Read the model definition and answer for the solid it produces. Units are mm, in the model's axes. Coordinates: 2 decimals unless noted, no trailing zeros. Loops run counter-clockwise (first coordinate to the right, second up) from the corner with the lowest first, then second, coordinate; pieces in that order, holes last.
from build123d import *

# Parameters (mm, degrees)
F0_R           = 12
F1_DEPTH       = 5
F2_R           = 21
F3_DEPTH       = 12.001
F3_DEPTH_BACK  = 12.001
F4_R           = 10.5
F5_DEPTH       = 6
F5_DEPTH_BACK  = 4
F6_SIZE        = 2
F8_D           = 4.5
F8_CSINK_D     = 10
F8_CSINK_ANGLE = 90


with BuildPart() as f1:
    # F0 (on Right) → F1 (new body)
    with BuildSketch(Plane.YZ):
        Circle(F0_R)
    extrude(amount=F1_DEPTH)

    # F2 (on Top) → F3 (cut, two sides)
    with BuildSketch(Plane.XY) as f3_sk:
        with Locations((-17, 0)):
            Circle(F2_R)
    extrude(amount=-F3_DEPTH, mode=Mode.SUBTRACT)
    extrude(f3_sk.sketch, amount=F3_DEPTH_BACK, mode=Mode.SUBTRACT)

    # F4 (on Right) → F5 (join, two sides)
    with BuildSketch(Plane.YZ) as f5_sk:
        Circle(F4_R)
    extrude(amount=-F5_DEPTH)
    extrude(f5_sk.sketch, amount=F5_DEPTH_BACK)

    # F6
    f6_edges = [f1.edges().sort_by_distance(p)[0] for p in [
        (-6, -10.5, 0),
    ]]
    chamfer(f6_edges, length=F6_SIZE)

    # F8 (through all)
    with Locations(Plane.YZ.offset(5)):
        with Locations((0, 0)):
            CounterSinkHole(F8_D / 2, F8_CSINK_D / 2, counter_sink_angle=F8_CSINK_ANGLE)


solid = f1.part
Q1. Determine the mould class of faces 1 (the face through (-0.83, -10.49, 0.46)), 2 (the face through (-6, 2, -2)), 3 (the face through (-1.93, 0.29, 2.23)) for opening direction Z: +Z half, -Z half, draft (parallel to the pull), parting line (faces both ways), or undercut.
Findings below:
face 1: parting line
face 2: draft
face 3: undercut
Q2. A cutting plane is placed at B-B (z = 0). Give the vertices of the cut face in (x, y), then the cut area to 3 significant figures.
Findings below:
outline: (-6, -8.5) - (-4, -10.5) - (1.19, -10.5) arc R21 cw to (0.23, -12) - (5, -12) - (5, -5) - (2.25, -2.25) - (-6, -2.25) - close; (-6, 2.25) - (2.25, 2.25) - (5, 5) - (5, 12) - (0.23, 12) arc R21 cw to (1.19, 10.5) - (-4, 10.5) - (-6, 8.5) - close
area: 183 mm2
Q3. Straight lines are drawn through the part: probe 1 along Y at (x, z) = (-3.5, 0); probe 2 along Z at (x, y) = (4.25, 1.5). For each, find the intervals that lie inside material, in ascending order.
Findings below:
probe 1: y = -10.5 to -2.25, 2.25 to 10.5
probe 2: z = -11.91 to -3.98, 3.98 to 11.91
Q4. A cutting plane is placed at C-C (x = -0.5). Give the vertices of the cut face in (y, z).
Findings below:
outline: circle Ø21 at (0, 0); hole circle Ø4.5 at (0, 0)
Q5. Flat-ended cylindrical pins translate along their axes: pin 1 Ø6 at (x, z) = (3.5, 6) entering from -Y; pin 2 Ø1.5 at (x, z) = (-2.5, -7.5) entering from +Y; pin 3 Ø4 at (x, y) = (-1, 2) entering from -Z. Find the tip coordinate at first contact, or state that the pin passes through.
Findings below:
pin 1: stops at y = -11.62
pin 2: stops at y = 8.04
pin 3: stops at z = -10.5
Q6. A cutting plane is placed at A-A (y = 0). Give the vertices of the cut face in (x, z), then the cut area to 3 significant figures.
Findings below:
outline: (-6, -8.5) - (-4, -10.5) - (4, -10.5) - (4, -12) - (5, -12) - (5, -5) - (2.25, -2.25) - (-6, -2.25) - close; (-6, 2.25) - (2.25, 2.25) - (5, 5) - (5, 12) - (4, 12) - (4, 10.5) - (-4, 10.5) - (-6, 8.5) - close
area: 173 mm2
